Can you work these out from the model? Positions are in its coordinate system, mm. Face numbers are marked on the shaded views. A direction names the side the tool comes from. Round coordinates to 2 decimals unless told otherwise and drop trailing zeros. Order: outer loops, then holes, each group sorted by start corner. A loop starts at its lowest first (then second) coordinate and runs counter-clockwise, first axis right, second up. Notation, with made-up numbers: (75.5, 18.25) -> (128.5, 18.25) arc R31 ccw to (128.5, 49.25) -> close; hole circle Ø7 at (45, -19.75). An arc over 180 degrees is marked (long way). One line per item, written item: value.
```python
from build123d import *

# Parameters (mm, degrees)
M16X1_5_GEWINDEBOHRUNG1_D           = 14.5
M16X1_5_GEWINDEBOHRUNG1_DEPTH       = 27.5
M16X1_5_GEWINDEBOHRUNG1_CSINK_D     = 16.05
M16X1_5_GEWINDEBOHRUNG1_CSINK_ANGLE = 90
M16X1_5_GEWINDEBOHRUNG1_TIP         = 4.356239488
FASE1_SIZE                          = 0.5


with BuildPart() as part:
    # Skizze1 → Rotation1 (revolve)
    with BuildSketch(Plane.XY, mode=Mode.PRIVATE) as rotation1_sk:
        Polygon((55, 4), (0, 4), (0, 8), (15, 8), (15, 10), (55, 10), align=None)
    revolve(rotation1_sk.sketch.rotate(Axis((0, 0, 0), (1, 0, 0)), 90), axis=Axis((0, 0, 0), (1, 0, 0)))

    # M16x1.5 Gewindebohrung1
    with Locations(Plane(origin=(55, 0, 0), x_dir=(0, 0, -1), z_dir=(1, 0, 0))):
        with Locations((0, 0)):
            CounterSinkHole(M16X1_5_GEWINDEBOHRUNG1_D / 2, M16X1_5_GEWINDEBOHRUNG1_CSINK_D / 2, depth=M16X1_5_GEWINDEBOHRUNG1_DEPTH, counter_sink_angle=M16X1_5_GEWINDEBOHRUNG1_CSINK_ANGLE)
            with Locations((0, 0, -(M16X1_5_GEWINDEBOHRUNG1_DEPTH + M16X1_5_GEWINDEBOHRUNG1_TIP / 2))):  # 118° drill point
                Cone(0, M16X1_5_GEWINDEBOHRUNG1_D / 2, M16X1_5_GEWINDEBOHRUNG1_TIP, mode=Mode.SUBTRACT)

    # Fase1
    fase1_edges = [part.edges().sort_by_distance(p)[0] for p in [
        (0, 0, -8),
    ]]
    chamfer(fase1_edges, length=FASE1_SIZE)

    # Skizze31 → Schnitt-Rotation1 (revolve, cut)
    with BuildSketch(Plane(origin=(15, 0, 0), x_dir=(1, 0, 0), z_dir=(0, 0, 1)), mode=Mode.PRIVATE) as schnitt_rotation1_sk:
        with BuildLine():
            Line((-5.366025404, 8), (-4.788675135, 7))
            ThreePointArc((-4.788675135, 7), (-4.422649731, 6.633974596), (-3.922649731, 6.5))
            Line((-3.922649731, 6.5), (-1, 6.5))
            ThreePointArc((-1, 6.5), (-0.292893219, 6.792893219), (0, 7.5))
            Line((0, 7.5), (0, 8))
            Line((0, 8), (-5.366025404, 8))
        make_face()
    revolve(schnitt_rotation1_sk.sketch.rotate(Axis((28.677186203, 0, 0), (-1, 0, 0)), 90), axis=Axis((28.677186203, 0, 0), (-1, 0, 0)), mode=Mode.SUBTRACT)


solid = part.part
```
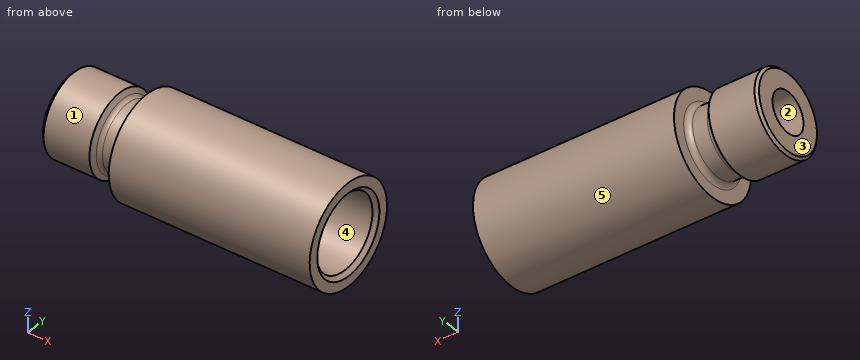
Q1. Will these pins go through, and if not, where does the flat tip stop? pin 1 Ø4 at (x, z) = (8, -4) entering from -Y; pin 2 Ø1 at (x, y) = (26.5, -7) entering from +Z; pin 3 Ø4 at (x, y) = (46.5, 3.5) entering from +Z.
Answers below:
pin 1: y = -7.75
pin 2: z = 7.6
pin 3: z = 9.89
Q2. I want a section at C-C on x = 50.5. List the corners of the cut face in (y, z) for me.
Answers below:
outline: circle Ø20 at (0, 0); hole circle Ø14.5 at (0, 0)
Q3. On a 3-axis mill with a long thin cutter (end or side, diameter ignored), from which of +Z, -Z, +X, -X, +Y, -Y can I reach the whole of each face in a straight line? I mean the marked faces 4 and 5. Say none if no direction works.
Answers below:
face 4: +X
face 5: +X, -X
Q4. I want a section at A-A on z = 0. List the corners of the cut face in (x, y) for me (3 decimals), plus the area to 3 significant figures.
Answers below:
outline: (0, -7.5) -> (0.5, -8) -> (9.634, -8) -> (10.211, -7) arc R1 cw to (11.077, -6.5) -> (14, -6.5) arc R1 cw to (15, -7.5) -> (15, -10) -> (55, -10) -> (55, -8.025) -> (54.225, -7.25) -> (27.5, -7.25) -> (25.547, -4) -> (0, -4) -> close; (0, 4) -> (25.547, 4) -> (27.5, 7.25) -> (54.225, 7.25) -> (55, 8.025) -> (55, 10) -> (15, 10) -> (15, 7.5) arc R1 cw to (14, 6.5) -> (11.077, 6.5) arc R1 cw to (10.211, 7) -> (9.634, 8) -> (0.5, 8) -> (0, 7.5) -> close
area: 400 mm^2
Q5. Please list where these lines run through material, in increasing order: line 1 along Y through (x, z) = (5.75, 0); line 2 along X through (y, z) = (7.5, 5.25); line 3 along Y through (x, z) = (16, 0).
Answers below:
line 1: -8 to -4, 4 to 8
line 2: 15 to 55
line 3: -10 to -4, 4 to 10
Q6. We'd pull the mould along Y, two halves only. Please class the marked faces 1, 2 and 3: released by +Y, released by -Y, zero draft, split by the parting line, or undercut.
Answers below:
face 1: split by the parting line
face 2: undercut
face 3: zero draft
